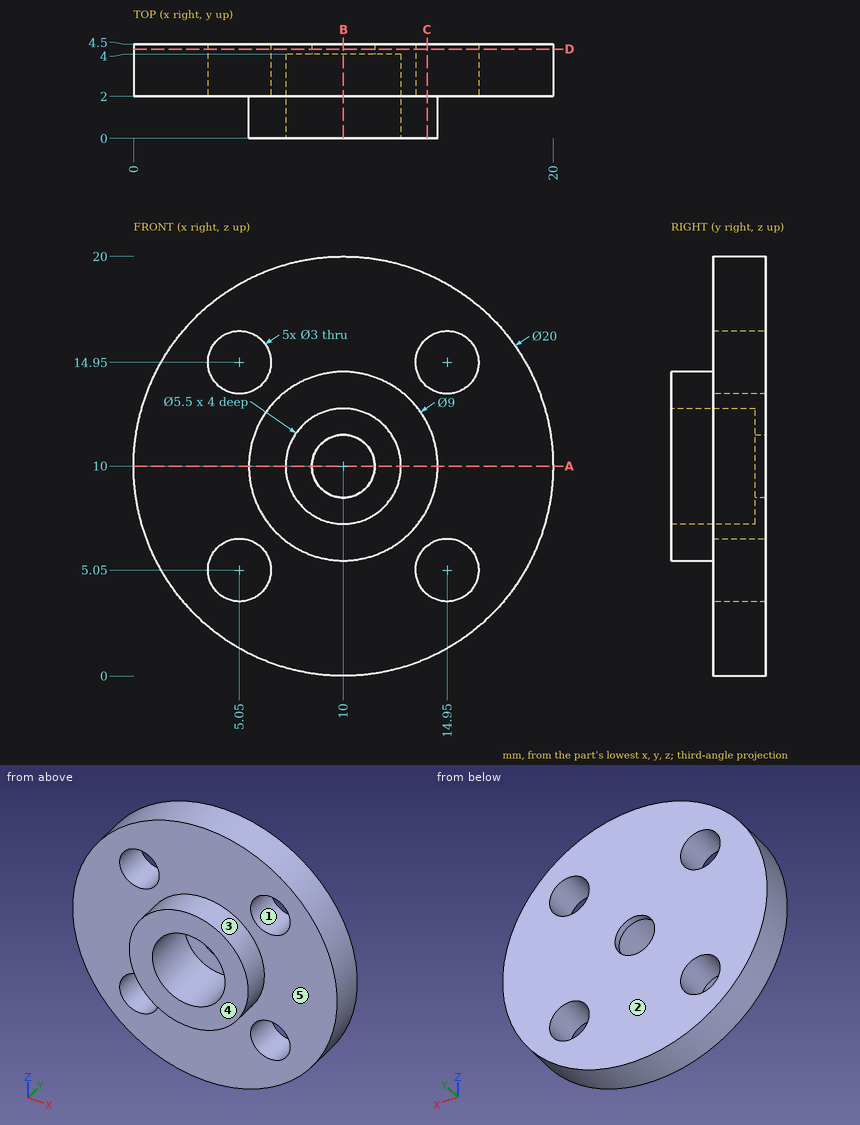
Verification items for this drawing (mm, ordinates from the low corner). A direction names the side the tool comes from. Coordinates: 2 decimals unless noted, no trailing zeros. Write each loop counter-clockwise with the first axis right and the second up, starting at its lowest first coordinate (ties: lowest second). Pieces come first, ordered by that corner, then holes. Notation, with made-up numbers: M 20,-39 L 74,-39 A8 cw 74,-25 Z; hole C 79.5,-6.5 d2. An arc over 180 degrees is marked long. Answer as a JSON object with one key per item and string values. Group by question number.
(1) Release check for a two-part mould opening along Z. For the marked faces 1, 2 and 3 record: +Z half, -Z half, draft (parallel to the pull), parting line (faces both ways), or undercut.
(2) Gauge pin test, flat ends, axial feed: pin 1 (2 mm diameter, centred on x = 11.5, z = 4.5, fed in from -Y); pin 2 (2 mm diameter, centred on y = 3, z = 7, fed in from -X); pin 3 (2 mm diameter, centred on y = 2, z = 16.5, fed in from +X). Record the tip position at first contact, or that the pin passes through.
(3) Cross-section at D-D, the plane y = 4.25. Record the cut outline in (x, z).
(4) Cross-section at C-C, the plane x = 14. Record the cut outline in (y, z) (1 decimal).
(5) Material ranges on line 1 (X direction, y = 4.3, z = 10); line 2 (X direction, y = 2.9, z = 4); line 3 (Z direction, x = 5, y = 3.6), recorded low to high.
(6) Cross-section at A-A, the plane z = 10. Record the cut outline in (x, y), and give its area (3 significant figures).
(7) Cross-section at B-B, the plane x = 10. Record the cut outline in (y, z), and give its area (3 significant figures).
(8) Tool access check on the marked faces 4 and 5. Record the directions out of +Z, -Z, +X, -X, +Y, -Y that give a thin tool (end or side, any length) a straight path to the whole face; none if there is none.
Reply:
{
 "1": {"face 1": "undercut", "face 2": "draft", "face 3": "parting line"},
 "2": {"pin 1": "y = 2", "pin 2": "x = 0.2", "pin 3": "x = 18.35"},
 "3": {"outline": "C 10,10 d20; hole C 5.05,5.05 d3; hole C 5.05,14.95 d3; hole C 10,10 d3; hole C 14.95,5.05 d3; hole C 14.95,14.95 d3"},
 "4": {"outline": "M 0,7.9 L 2,7.9 L 2,6.2 L 4.5,6.2 L 4.5,13.8 L 2,13.8 L 2,12.1 L 0,12.1 Z; M 2,0.8 L 4.5,0.8 L 4.5,3.9 L 2,3.9 Z; M 2,16.1 L 4.5,16.1 L 4.5,19.2 L 2,19.2 Z"},
 "5": {"line 1": "0 to 8.5, 11.5 to 20", "line 2": "2 to 3.98, 6.12 to 13.88, 16.02 to 18", "line 3": "1.34 to 3.55, 6.55 to 13.45, 16.45 to 18.66"},
 "6": {"outline": "M 0,2 L 5.5,2 L 5.5,0 L 7.25,0 L 7.25,4 L 8.5,4 L 8.5,4.5 L 0,4.5 Z; M 11.5,4 L 12.75,4 L 12.75,0 L 14.5,0 L 14.5,2 L 20,2 L 20,4.5 L 11.5,4.5 Z", "area": "44.5 mm²"},
 "7": {"outline": "M 0,5.5 L 2,5.5 L 2,0 L 4.5,0 L 4.5,8.5 L 4,8.5 L 4,7.25 L 0,7.25 Z; M 0,12.75 L 4,12.75 L 4,11.5 L 4.5,11.5 L 4.5,20 L 2,20 L 2,14.5 L 0,14.5 Z", "area": "44.5 mm²"},
 "8": {"face 4": "+Z, -Z, +X, -X, -Y", "face 5": "-Y"}
}
